```python
from build123d import *

# Parameters (mm, degrees)
SKETCH_1_R      = 3
EXTRUDE_1_DEPTH = 3
SKETCH_1_3_R    = 3
SKETCH_1_3_R_2  = 1.7
EXTRUDE_2_DEPTH = 10
CHAMFER_1_SIZE  = 1.4


with BuildPart() as part:
    # Sketch 1 → Extrude 1 (new body)
    with BuildSketch(Plane.XY):
        with BuildLine():
            Line((-7.5, 15), (7.5, 15))
            ThreePointArc((7.5, 15), (22.5, 0), (7.5, -15))
            Line((7.5, -15), (-7.5, -15))
            ThreePointArc((-7.5, -15), (-22.5, 0), (-7.5, 15))
        make_face()
        with Locations((-10, 0)):
            Circle(SKETCH_1_R, mode=Mode.SUBTRACT)
        with Locations((10, 0)):
            Circle(SKETCH_1_R, mode=Mode.SUBTRACT)
    extrude(amount=EXTRUDE_1_DEPTH)

    # Sketch 1_3 → Extrude 2 (add)
    # profile 1 of 2: a face of its own
    with BuildSketch(Plane.XY):
        with Locations((-10, 0)):
            Circle(SKETCH_1_3_R)
        with Locations((-10, 0)):
            Circle(SKETCH_1_3_R_2, mode=Mode.SUBTRACT)
    # profile 2 of 2: a face of its own
    with BuildSketch(Plane.XY):
        with Locations((10, 0)):
            Circle(SKETCH_1_3_R)
        with Locations((10, 0)):
            Circle(SKETCH_1_3_R_2, mode=Mode.SUBTRACT)
    extrude(amount=EXTRUDE_2_DEPTH)

    # Chamfer 1
    chamfer_1_edges = [part.edges().sort_by_distance(p)[0] for p in [
        (-11.7, 0, 0),
        (8.3, 0, 0),
    ]]
    chamfer(chamfer_1_edges, length=CHAMFER_1_SIZE)


solid = part.part
```
For this review, take the finished solid that the model builds, in its own axes (mm). A direction names the side the tool comes from. Round coordinates to 2 decimals unless told otherwise and drop trailing zeros. Write each loop counter-clockwise with the first axis right and the second up, starting at its lowest first coordinate (ties: lowest second). Pieces come first, ordered by that corner, then holes.
1) Insertion check: pin 1 Ø3 at (y, z) = (-1, 5.5) entering from -X; pin 2 Ø5.5 at (x, y) = (-10, 0) entering from -Z; pin 3 Ø4 at (y, z) = (0.5, 5.5) entering from +X. Each pin has a flat end and moves straight along its axis. Give the tip position at first contact, or say it passes through.
Answer below:
pin 1: stops at x = -13
pin 2: stops at z = 0.35
pin 3: stops at x = 13
2) Take a section at A-A on y = 0. Give the boundary of the cut face in (x, z).
Answer below:
outline: (-22.5, 0) - (-13.1, 0) - (-11.7, 1.4) - (-11.7, 10) - (-13, 10) - (-13, 3) - (-22.5, 3) - close; (-8.3, 1.4) - (-6.9, 0) - (6.9, 0) - (8.3, 1.4) - (8.3, 10) - (7, 10) - (7, 3) - (-7, 3) - (-7, 10) - (-8.3, 10) - close; (11.7, 1.4) - (13.1, 0) - (22.5, 0) - (22.5, 3) - (13, 3) - (13, 10) - (11.7, 10) - close
3) Take a section at D-D on z = 9. Give the boundary of the cut face in (x, y).
Answer below:
outline: circle Ø6 at (-10, 0); circle Ø6 at (10, 0); hole circle Ø3.4 at (-10, 0); hole circle Ø3.4 at (10, 0)
4) Take a section at B-B on x = -10. Give the boundary of the cut face in (y, z), then the cut area to 3 significant figures.
Answer below:
outline: (-14.79, 0) - (-3.1, 0) - (-1.7, 1.4) - (-1.7, 10) - (-3, 10) - (-3, 3) - (-14.79, 3) - close; (1.7, 1.4) - (3.1, 0) - (14.79, 0) - (14.79, 3) - (3, 3) - (3, 10) - (1.7, 10) - close
area: 94.8 mm2
5) Machinability: for faces 4 (the face through (12.77, -1.15, 6.45)), 5 (the face through (-8, 0, 10)), which of the approach directions +Z, -Z, +X, -X, +Y, -Y give a long, thin tool a straight path to every point of the face, cutting with its end or side? Answer none if there is none.
Answer below:
face 4: +Z
face 5: +Z, +X, -X, +Y, -Y
6) For line 1 along Y through (x, z) = (-10, 6.5); line 2 along X through (y, z) = (0, 1); line 3 along Z through (x, y) = (8, -10), list the stretches that pass through material, from the lowest coordinate up.
Answer below:
line 1: y = -3 to -1.7, 1.7 to 3
line 2: x = -22.5 to -12.1, -7.9 to 7.9, 12.1 to 22.5
line 3: z = 0 to 3
7) Take a section at C-C on z = 0.75. Give the boundary of the cut face in (x, y).
Answer below:
outline: (-7.5, -15) - (7.5, -15) arc R15 ccw to (7.5, 15) - (-7.5, 15) arc R15 ccw to start; hole circle Ø4.7 at (-10, 0); hole circle Ø4.7 at (10, 0)
8) Mouldability with a two-part tool opening along Y and no side actions: class faces 1 (the face through (0, 0, 3)), 2 (the face through (9.63, -1.66, 5.64)), 3 (the face through (-12.4, -1.8, 6.5)) as +Y half, -Y half, draft (parallel to the pull), parting line (faces both ways), or undercut.
Answer below:
face 1: draft
face 2: undercut
face 3: parting line
